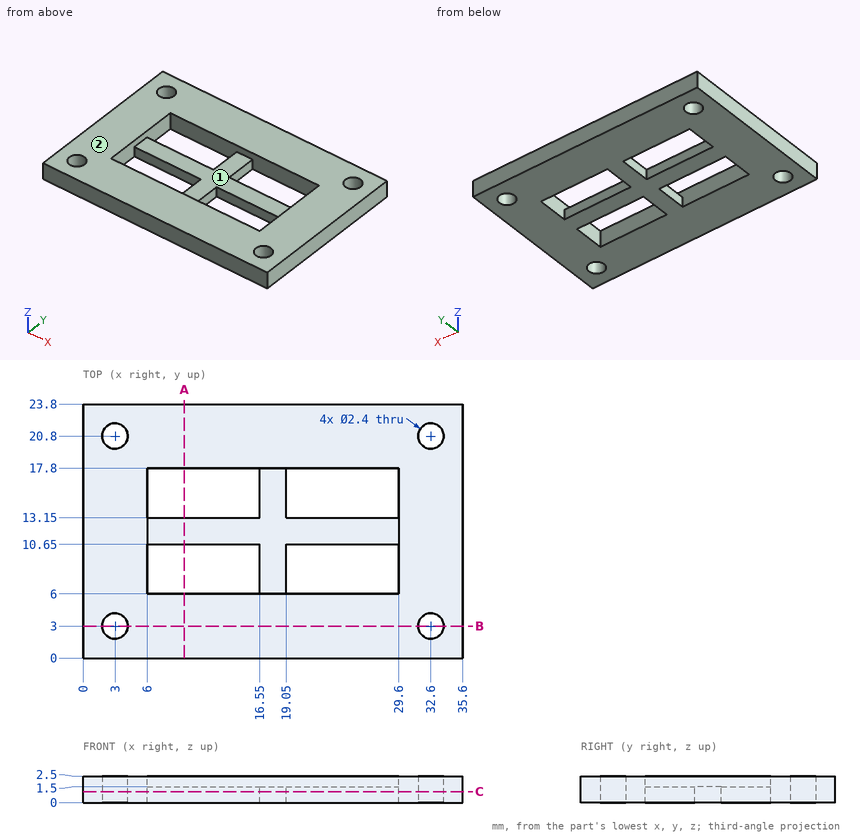
Geometry check sheet. Reference: drawing and pictorial views, mm from the part's lowest x, y, z. Give positions to 0.01 mm unless a question says otherwise; leave off trailing zeros. Order: outer loops, then holes, each group sorted by start corner. A loop starts at its lowest first (then second) coordinate and runs counter-clockwise, first axis right, second up. Notation, with made-up numbers: (19.5, 84) - (73.5, 84) arc R16 cw to (73.5, 101) - close; hole circle Ø2 at (17, -12). An arc over 180 degrees is marked (long way). Use one line per item in the form item = value.
1) Material ranges on probe 1 along Y at (x, z) = (21, 0.95); probe 2 along X at (y, z) = (20.75, 1.4); probe 3 along X at (y, z) = (9.75, 1.1), recorded low to high. Write a range as from..to.
Working result:
probe_1 = 0..6, 10.65..13.15, 17.8..23.8
probe_2 = 0..1.8, 4.2..31.4, 33.8..35.6
probe_3 = 0..6, 16.55..19.05, 29.6..35.6
2) Sectioned sample at A-A (x = 9.5). Record the boundary of the cut face in (y, z), and give its area (4 significant figures).
Working result:
outline = (0, 0) - (6, 0) - (6, 2.5) - (0, 2.5) - close; (10.65, 0) - (13.15, 0) - (13.15, 1.5) - (10.65, 1.5) - close; (17.8, 0) - (23.8, 0) - (23.8, 2.5) - (17.8, 2.5) - close
area = 33.75 mm^2
3) Sectioned sample at C-C (z = 1.05). Count the separate pieces of the cut face and the enclosed holes in it, and give its area (3 significant figures).
Working result:
separate_pieces = 1
enclosed_holes = 8
area = 633 mm^2
4) Draft check along X on the marked faces 1 and 2. Enter one of: released by +X, released by -X, zero draft, split by the parting line, or undercut.
Working result:
face_1 = undercut
face_2 = zero draft
5) Sectioned sample at B-B (y = 3). Record the boundary of the cut face in (x, z), and give its area (3 significant figures).
Working result:
outline = (0, 0) - (1.8, 0) - (1.8, 2.5) - (0, 2.5) - close; (4.2, 0) - (31.4, 0) - (31.4, 2.5) - (4.2, 2.5) - close; (33.8, 0) - (35.6, 0) - (35.6, 2.5) - (33.8, 2.5) - close
area = 77.0 mm^2
6) Depth check by flat-ended pin: pin 1 Ø6 at (x, y) = (12.5, 10) entering from +Z. Enter the tip coordinate at first touch or a pass-through.
Working result:
pin_1 = 1.5
